Design review of the part built by this model. Coordinates are the model's own, in mm. A direction names the side the tool comes from. Round coordinates to 2 decimals unless told otherwise and drop trailing zeros. Loops run counter-clockwise (first coordinate to the right, second up) from the corner with the lowest first, then second, coordinate; pieces in that order, holes last. Notation, with made-up numbers: (-27, -38.5) - (-1, -38.5) arc R16 cw to (-1, -30.5) - close; hole circle Ø3 at (-39, 76). An arc over 180 degrees is marked (long way). One line per question, with ' | ' between items. Start each with the question number.
from build123d import *

# Parameters (mm, degrees)
CROQUIS1_W              = 200
CROQUIS1_H              = 130
SALIENTE_EXTRUIR1_DEPTH = 3
CROQUIS2_W              = 5
CROQUIS2_H              = 5
CROQUIS2_H_2            = 120
CROQUIS2_W_2            = 190
SALIENTE_EXTRUIR2_DEPTH = 67
CROQUIS3_W              = 190
CROQUIS3_H              = 15
CORTAR_EXTRUIR1_DEPTH   = 5
CROQUIS4_W              = 196
CROQUIS4_H              = 3.05
CORTAR_EXTRUIR2_DEPTH   = 126
CROQUIS7_W              = 190
CROQUIS7_H              = 3
CORTAR_EXTRUIR3_DEPTH   = 5
CROQUIS8_R              = 2
CORTAR_EXTRUIR4_DEPTH   = 5


with BuildPart() as part:
    # Croquis1 → Saliente-Extruir1 (new body)
    with BuildSketch(Plane(origin=(0, 0, 0), x_dir=(1, 0, 0), z_dir=(0, 1, 0))):
        Rectangle(CROQUIS1_W, CROQUIS1_H)
    extrude(amount=SALIENTE_EXTRUIR1_DEPTH)

    # Croquis2 → Saliente-Extruir2 (add)
    with BuildSketch(Plane(origin=(0, 3, 0), x_dir=(1, 0, 0), z_dir=(0, 1, 0))):
        with Locations((-97.5, 62.5)):
            Rectangle(CROQUIS2_W, CROQUIS2_H)
        with Locations((-97.5, 0)):
            Rectangle(CROQUIS2_W, CROQUIS2_H_2)
        with Locations((0, 62.5)):
            Rectangle(CROQUIS2_W_2, CROQUIS2_H)
        with Locations((97.5, 62.5)):
            Rectangle(CROQUIS2_W, CROQUIS2_H)
        with Locations((-97.5, -62.5)):
            Rectangle(CROQUIS2_W, CROQUIS2_H)
        with Locations((97.5, 0)):
            Rectangle(CROQUIS2_W, CROQUIS2_H_2)
        with Locations((0, -62.5)):
            Rectangle(CROQUIS2_W_2, CROQUIS2_H)
        with Locations((97.5, -62.5)):
            Rectangle(CROQUIS2_W, CROQUIS2_H)
    extrude(amount=SALIENTE_EXTRUIR2_DEPTH)

    # Croquis3 → Cortar-Extruir1 (cut)
    with BuildSketch(Plane.XY.offset(65)):
        with Locations((0, 10.5)):
            Rectangle(CROQUIS3_W, CROQUIS3_H)
    extrude(amount=-CORTAR_EXTRUIR1_DEPTH, mode=Mode.SUBTRACT)

    # Croquis4 → Cortar-Extruir2 (cut)
    with BuildSketch(Plane.XY.offset(65)):
        with Locations((0, 65.475)):
            Rectangle(CROQUIS4_W, CROQUIS4_H)
    extrude(amount=-CORTAR_EXTRUIR2_DEPTH, mode=Mode.SUBTRACT)

    # Croquis7 → Cortar-Extruir3 (cut)
    with BuildSketch(Plane(origin=(0, 0, 60), x_dir=(-1, 0, 0), z_dir=(0, 0, -1))):
        with Locations((0, 68.5)):
            Rectangle(CROQUIS7_W, CROQUIS7_H)
    extrude(amount=-CORTAR_EXTRUIR3_DEPTH, mode=Mode.SUBTRACT)

    # Croquis8 → Cortar-Extruir4 (cut)
    with BuildSketch(Plane(origin=(0, 0, -65), x_dir=(-1, 0, 0), z_dir=(0, 0, -1))):
        with Locations((-35, 7.5)):
            Circle(CROQUIS8_R)
    extrude(amount=-CORTAR_EXTRUIR4_DEPTH, mode=Mode.SUBTRACT)


solid = part.part
1. Clearance check with flat-ended pins moving along their axes: P1, Ø5, axis at x = 47, z = 7.5, coming from the +Y side; P2, Ø3.5, axis at x = 14.5, y = 69, coming from the +Z side; P3, Ø3.5, axis at x = -13.5, y = 65.5, coming from the +Z side. State where each tip first meets the part, or that it passes through.
2. Take a section at A-A, the plane x = -85.5. Give the boundary of the cut face in (y, z).
3. Take a section at C-C, the plane x = 35. Give the boundary of the cut face in (y, z).
4. Take a section at B-B, the plane y = 7.5. Give the boundary of the cut face in (x, z), then the cut area to 3 significant figures.
5. Machinability: for faces 1 (the face through (1, 35, -65)), 2 (the face through (-1, 41, 60)), which of the approach directions +Z, -Z, +X, -X, +Y, -Y give a long, thin tool a straight path to every point of the face, cutting with its end or side? Answer none if there is none.
6. To check wall thickness, follow line 1 along X through (y, z) = (51, -44); line 2 along Z through (x, y) = (-49, 49); line 3 along Y through (x, z) = (35, -62). State the ranges of each line that lie inside material, in increasing order.
7. Take a section at D-D, the plane y = 25. Give the boundary of the cut face in (x, z).
8. The part is to be moulded in two halves that separate along X. For faces 3 (the face through (-1, 42, 65)), 4 (the face through (-100, 35, -1)), 5 (the face through (-1, 18, 63)), say which applies: pulls with the +X half, pulls with the -X half, needs draft (parallel to the pull), parting line crosses it, or undercut.
Answer list:
1) P1: stops at y = 3 | P2: stops at z = -60 | P3: stops at z = 65
2) outline: (0, -65) - (70, -65) - (70, -60) - (67, -60) - (67, -61) - (63.95, -61) - (63.95, -60) - (3, -60) - (3, 65) - (0, 65) - close; (18, 60) - (63.95, 60) - (63.95, 65) - (18, 65) - close
3) outline: (0, -65) - (5.5, -65) - (5.5, -60) - (3, -60) - (3, 65) - (0, 65) - close; (9.5, -65) - (70, -65) - (70, -60) - (67, -60) - (67, -61) - (63.95, -61) - (63.95, -60) - (9.5, -60) - close; (18, 60) - (63.95, 60) - (63.95, 65) - (18, 65) - close
4) outline: (-100, -65) - (33, -65) - (33, -60) - (-95, -60) - (-95, 65) - (-100, 65) - close; (37, -65) - (100, -65) - (100, 65) - (95, 65) - (95, -60) - (37, -60) - close | area: 2,230 mm²
5) face 1: -Z, +X, -X, +Y, -Y | face 2: +Y
6) line 1: x = -100 to -95, 95 to 100 | line 2: z = -65 to -60, 60 to 65 | line 3: y = 0 to 5.5, 9.5 to 70
7) outline: (-100, -65) - (100, -65) - (100, 65) - (-100, 65) - close; hole (-95, -60) - (95, -60) - (95, 60) - (-95, 60) - close
8) face 3: needs draft | face 4: pulls with the -X half | face 5: undercut
